Study the drawing (mm; zero at the part's minimum x, y, z) and answer. A direction names the side the tool comes from. Round coordinates to 2 decimals unless told otherwise and drop trailing zeros. Write each loop counter-clockwise with the first axis right and the second up, starting at its lowest first coordinate (ties: lowest second). Pieces come first, ordered by that corner, then holes.
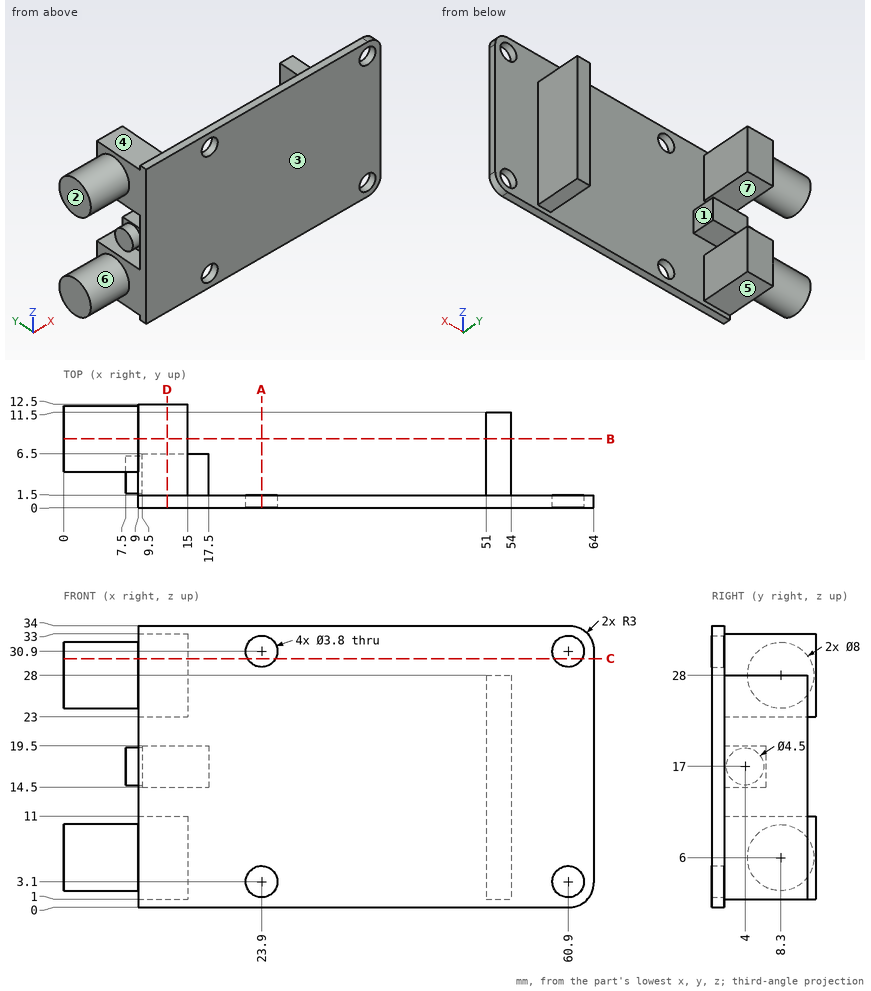
1. For a pull along X with two mould halves and no side action, classify the marked faces 1, 2 and 3 as released by +X, released by -X, zero draft, split by the parting line, or undercut.
Geometry says:
face 1: undercut
face 2: released by -X
face 3: zero draft
2. Straight lines are drawn through the part: line 1 along Z through (x, y) = (60.9, 0.95); line 2 along X through (y, z) = (4.5, 19); line 3 along X through (y, z) = (9, 5). For each, find the intervals that lie inside material, in ascending order.
Geometry says:
line 1: z = 0 to 1.2, 5 to 29, 32.8 to 34
line 2: x = 7.5 to 17.5, 51 to 54
line 3: x = 0 to 15, 51 to 54
3. Section C-C on z = 30 is taken. Determine the outline of the cut face in (x, y), plus the area to 3 significant figures.
Geometry says:
outline: (0, 4.84) - (9, 4.84) - (9, 0) - (22.23, 0) - (22.23, 1.5) - (15, 1.5) - (15, 12.5) - (9, 12.5) - (9, 11.76) - (0, 11.76) - close; (25.57, 0) - (59.23, 0) - (59.23, 1.5) - (25.57, 1.5) - close; (62.57, 0) - (64, 0) - (64, 1.5) - (62.57, 1.5) - close
area: 201 mm2
4. Section A-A on x = 23.9 is taken. Determine the outline of the cut face in (y, z), plus the area to 3 significant figures.
Geometry says:
outline: (0, 0) - (1.5, 0) - (1.5, 1.2) - (0, 1.2) - close; (0, 5) - (1.5, 5) - (1.5, 29) - (0, 29) - close; (0, 32.8) - (1.5, 32.8) - (1.5, 34) - (0, 34) - close
area: 39.6 mm2
5. Given pin 1 (3.5 mm diameter, centred on x = 23.9, z = 30.9, fed in from -Y) (3 decimals); pin 2 (0.9 mm diameter, centred on x = 53, y = 7.5, fed in from +Z); pin 3 (2.5 mm diameter, centred on x = 52.5, z = 10, fed in from +Y); pin 4 (1.5 mm diameter, centred on y = 5.5, z = 29.5, fed in from +X), each flat-ended and moving along its own axis, determine where each tip first touches the part or whether it passes through.
Geometry says:
pin 1: passes through
pin 2: stops at z = 28
pin 3: stops at y = 11.5
pin 4: stops at x = 15
6. A tool of negligible diameter and unlimited length cuts with its end or side. For the marked faces 4, 5, 6 and 7, from which of +Z, -Z, +X, -X, +Y, -Y can it reach the whole face along a straight path? Write none if from no direction.
Geometry says:
face 4: +Z, +X, -X, +Y
face 5: -Z, +X, -X, +Y
face 6: -X
face 7: -X, +Y
7. Section B-B on y = 8.3 is taken. Determine the outline of the cut face in (x, z).
Geometry says:
outline: (0, 2) - (9, 2) - (9, 1) - (15, 1) - (15, 11) - (9, 11) - (9, 10) - (0, 10) - close; (0, 24) - (9, 24) - (9, 23) - (15, 23) - (15, 33) - (9, 33) - (9, 32) - (0, 32) - close; (51, 1) - (54, 1) - (54, 28) - (51, 28) - close
8. Section D-D on x = 12.5 is taken. Determine the outline of the cut face in (y, z), plus the area to 3 significant figures.
Geometry says:
outline: (0, 0) - (1.5, 0) - (1.5, 1) - (12.5, 1) - (12.5, 11) - (1.5, 11) - (1.5, 14.5) - (6.5, 14.5) - (6.5, 19.5) - (1.5, 19.5) - (1.5, 23) - (12.5, 23) - (12.5, 33) - (1.5, 33) - (1.5, 34) - (0, 34) - close
area: 296 mm2
